Source: CAD feature listing. Evaluate the final solid. Frame: model axes, mm. Round coordinates to 2 decimals unless told otherwise and drop trailing zeros. Write each loop counter-clockwise with the first axis right and the second up, starting at its lowest first coordinate (ties: lowest second). Pieces come first, ordered by that corner, then holes. Notation, with made-up numbers: M 75,0.25 L 130,0.25 A17 ccw 130,24.25 Z; hole C -24.75,-1 d5. An arc over 180 degrees is marked long. Answer in a Markdown table with one row per item.
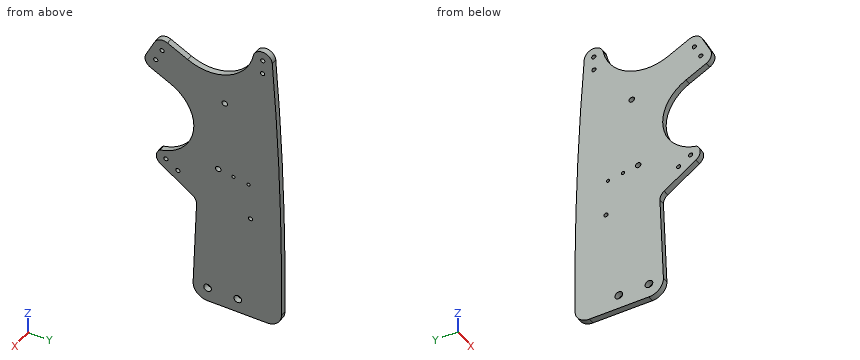
from build123d import *

# Parameters (mm, degrees)
SKETCH2_R           = 1.7272
SKETCH2_R_2         = 2.25425
SKETCH2_R_3         = 1.352550022
SKETCH2_R_4         = 3.175
BOSS_EXTRUDE1_DEPTH = 4.953


with BuildPart() as part:
    # Sketch2 → Boss-Extrude1 (new body)
    with BuildSketch(Plane(origin=(0, 0, 0), x_dir=(0, 0, -1), z_dir=(1, 0, 0))):
        with BuildLine():
            Line((-268, 33.638045694), (-268, -15.648345659))
            ThreePointArc((-268, -15.648345659), (-271.681104191, -24.296812143), (-280.46599542, -27.639294256))
            Line((-280.46599542, -27.639294256), (-354.369890721, -24.767221505))
            ThreePointArc((-354.369890721, -24.767221505), (-358.291047411, -25.622255962), (-361.303569715, -28.273908856))
            Line((-361.303569715, -28.273908856), (-379.165898581, -54.637880239))
            ThreePointArc((-379.165898581, -54.637880239), (-385.420991101, -58.116858889), (-391.93317504, -55.146852962))
            ThreePointArc((-391.93317504, -55.146852962), (-421.403553341, -27.354673474), (-457.218589828, -46.280623895))
            Line((-457.218589828, -46.280623895), (-465.626255558, -63.10041384))
            ThreePointArc((-465.626255558, -63.10041384), (-470.251425545, -67.112661913), (-476.359002427, -66.679260672))
            Line((-476.359002427, -66.679260672), (-490.566300389, -59.577494681))
            ThreePointArc((-490.566300389, -59.577494681), (-494.578548462, -54.952324694), (-494.145147221, -48.844747812))
            Line((-494.145147221, -48.844747812), (-485.73748149, -32.024957868))
            ThreePointArc((-485.73748149, -32.024957868), (-485.593767218, 1.721364638), (-512.325819935, 22.318264742))
            ThreePointArc((-512.325819935, 22.318264742), (-518.692977578, 30.592013537), (-511.35460422, 38.017906886))
            ThreePointArc((-511.35460422, 38.017906886), (-395.707987807, 44.184774715), (-279.906177735, 45.637678913))
            ThreePointArc((-279.906177735, 45.637678913), (-271.481612031, 42.090090796), (-268, 33.638045694))
        make_face()
        with Locations((-379.006254083, -40.251135649)):
            Circle(SKETCH2_R, mode=Mode.SUBTRACT)
        with Locations((-510.7706223, 30.101918548)):
            Circle(SKETCH2_R, mode=Mode.SUBTRACT)
        with Locations((-457.75455229, -1.41718755)):
            Circle(SKETCH2_R_2, mode=Mode.SUBTRACT)
        with Locations((-394.480328138, -6.767192974)):
            Circle(SKETCH2_R_2, mode=Mode.SUBTRACT)
        with Locations((-359.276554144, 19.928216477)):
            Circle(SKETCH2_R, mode=Mode.SUBTRACT)
        with Locations((-385.737171654, -50.185658721)):
            Circle(SKETCH2_R, mode=Mode.SUBTRACT)
        with Locations((-390.419716853, 18.306128226)):
            Circle(SKETCH2_R_3, mode=Mode.SUBTRACT)
        with Locations((-392.450022496, 5.769467626)):
            Circle(SKETCH2_R_3, mode=Mode.SUBTRACT)
        with Locations((-498.771367049, 29.968227033)):
            Circle(SKETCH2_R, mode=Mode.SUBTRACT)
        with Locations((-474.518853752, -58.65529334)):
            Circle(SKETCH2_R, mode=Mode.SUBTRACT)
        with Locations((-485.252549027, -53.289868312)):
            Circle(SKETCH2_R, mode=Mode.SUBTRACT)
        with Locations((-280, -15.648345659)):
            Circle(SKETCH2_R_4, mode=Mode.SUBTRACT)
        with Locations((-280, 9.351654341)):
            Circle(SKETCH2_R_4, mode=Mode.SUBTRACT)
    extrude(amount=BOSS_EXTRUDE1_DEPTH)


solid = part.part
Q1. Section B-B (z = 329). Return loops of the section in (x, y), and give its area (3 significant figures).
Solutions:
| item | result |
|---|---|
| outline | M 0,-25.75 L 4.95,-25.75 L 4.95,45.6 L 0,45.6 Z |
| area | 353 mm2 |
Q2. Section A-A (x = 1.4). State how many separate pieces and enclosed holes the cut face has, and give its area (3 significant figures).
Solutions:
| item | result |
|---|---|
| separate pieces | 1 |
| enclosed holes | 13 |
| area | 18,000 mm2 |
Q3. Material intervals for probe 1 along Y at (x, z) = (2.05, 280); probe 2 along Z at (x, y) = (4, -40.5); probe 3 along Y at (x, z) = (3.9, 395), sorted ascending.
Solutions:
| item | result |
|---|---|
| probe 1 | y = -27.65 to -18.82, -12.47 to 6.18, 12.53 to 45.64 |
| probe 2 | z = 369.59 to 377.3, 380.72 to 398.59, 453.58 to 489.97 |
| probe 3 | y = -46.19 to -8.96, -4.57 to 44.21 |
Q4. Contact query for flat-ended pins moving along their axis: pin 1 Ø4.5 at (y, z) = (-53.29, 485.25) entering from +X; pin 2 Ø2 at (x, y) = (3.5, -44) entering from +Z. Output: stop coordinate, or through.
Solutions:
| item | result |
|---|---|
| pin 1 | stops at x = 4.95 |
| pin 2 | stops at z = 492.22 |
Q5. Section C-C (z = 450.5). Return loops of the section in (x, y).
Solutions:
| item | result |
|---|---|
| outline | M 0,-37.04 L 4.95,-37.04 L 4.95,41.85 L 0,41.85 Z |
